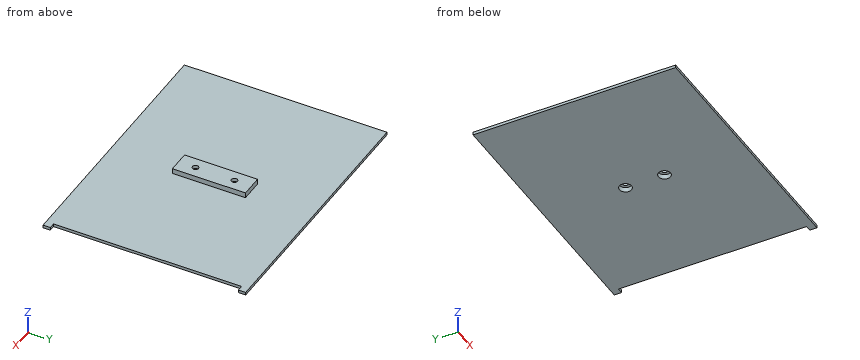
```python
from build123d import *

# Parameters (mm, degrees)
EXTRUDE_2_DEPTH     = 1.5
SKETCH_2_W          = 11.5
SKETCH_2_H          = 37.5
EXTRUDE_3_DEPTH     = 2.7
SKETCH_3_R          = 3.1
CUT_EXTRUDE_1_DEPTH = 2.5
SKETCH_4_R          = 1.55
CUT_EXTRUDE_2_DEPTH = 2.5


with BuildPart() as part:
    # Эскиз1 → Бобышка-Вытянуть2 (new body)
    with BuildSketch(Plane.XY):
        Polygon((-67, -52), (67, -52), (67, -48.25), (64, -48.25), (64, 48.25), (67, 48.25), (67, 52), (-67, 52), align=None)
    extrude(amount=EXTRUDE_2_DEPTH)

    # Эскиз2 → Бобышка-Вытянуть3 (add)
    with BuildSketch(Plane.XY.offset(1.5)):
        Rectangle(SKETCH_2_W, SKETCH_2_H)
    extrude(amount=EXTRUDE_3_DEPTH)

    # Эскиз3 → Вырез-Вытянуть1 (cut)
    with BuildSketch(Plane(origin=(0, 0, 0), x_dir=(-1, 0, 0), z_dir=(0, 0, -1))):
        with Locations((0, -10)):
            Circle(SKETCH_3_R)
        with Locations((0, 10)):
            Circle(SKETCH_3_R)
    extrude(amount=-CUT_EXTRUDE_1_DEPTH, mode=Mode.SUBTRACT)

    # Эскиз4 → Вырез-Вытянуть2 (cut)
    with BuildSketch(Plane(origin=(0, 0, 2.5), x_dir=(-1, 0, 0), z_dir=(0, 0, -1))):
        with Locations((0, -10)):
            Circle(SKETCH_4_R)
        with Locations((0, 10)):
            Circle(SKETCH_4_R)
    extrude(amount=-CUT_EXTRUDE_2_DEPTH, mode=Mode.SUBTRACT)


solid = part.part
```
Check sheet for the modelled part. Datum: model origin and axes. Units: mm. Round coordinates to 2 decimals unless told otherwise and drop trailing zeros. Order: outer loops, then holes, each group sorted by start corner. A loop starts at its lowest first (then second) coordinate and runs counter-clockwise, first axis right, second up. Notation, with made-up numbers: (-9.75, -31) -> (11.25, -31) arc R11 cw to (11.25, -16) -> close; hole circle Ø11 at (-12, -21.5). An arc over 180 degrees is marked (long way). One line per item, written item: value. Start each with the question number.
Q1. Cross-section at B-B (x = 0). Record the boundary of the cut face in (y, z).
Q2. Cross-section at D-D (x = 16.5). Record the boundary of the cut face in (y, z), and give its area (3 significant figures).
Q3. Gauge pin test, flat ends, axial feed: pin 1 Ø1.4 at (x, z) = (-1.5, 3.5) entering from -Y; pin 2 Ø2 at (x, z) = (-2.5, 3.5) entering from +Y; pin 3 Ø8 at (x, y) = (-45, 5) entering from +Z. Record the tip position at first contact, or that the pin passes through.
Q4. Thickness scan on line 1 (Y direction, x = 0, z = 3.1); line 2 (Y direction, x = 0, z = 0.8); line 3 (Z direction, x = 12, y = -19.5). Record the ranges inside material, lowest first.
Q5. Cross-section at C-C (z = 0.65). Record the boundary of the cut face in (x, y).
Q6. Cross-section at A-A (y = 10). Record the boundary of the cut face in (x, z), and give its area (3 significant figures).
Completed:
1. outline: (-52, 0) -> (-13.1, 0) -> (-13.1, 2.5) -> (-11.55, 2.5) -> (-11.55, 4.2) -> (-18.75, 4.2) -> (-18.75, 1.5) -> (-52, 1.5) -> close; (-8.45, 2.5) -> (-6.9, 2.5) -> (-6.9, 0) -> (6.9, 0) -> (6.9, 2.5) -> (8.45, 2.5) -> (8.45, 4.2) -> (-8.45, 4.2) -> close; (11.55, 2.5) -> (13.1, 2.5) -> (13.1, 0) -> (52, 0) -> (52, 1.5) -> (18.75, 1.5) -> (18.75, 4.2) -> (11.55, 4.2) -> close
2. outline: (-52, 0) -> (52, 0) -> (52, 1.5) -> (-52, 1.5) -> close
2. area: 156 mm²
3. pin 1: stops at y = -18.75
3. pin 2: stops at y = 18.75
3. pin 3: stops at z = 1.5
4. line 1: y = -18.75 to -11.55, -8.45 to 8.45, 11.55 to 18.75
4. line 2: y = -52 to -13.1, -6.9 to 6.9, 13.1 to 52
4. line 3: z = 0 to 1.5
5. outline: (-67, -52) -> (67, -52) -> (67, -48.25) -> (64, -48.25) -> (64, 48.25) -> (67, 48.25) -> (67, 52) -> (-67, 52) -> close; hole circle Ø6.2 at (0, -10); hole circle Ø6.2 at (0, 10)
6. outline: (-67, 0) -> (-3.1, 0) -> (-3.1, 2.5) -> (-1.55, 2.5) -> (-1.55, 4.2) -> (-5.75, 4.2) -> (-5.75, 1.5) -> (-67, 1.5) -> close; (1.55, 2.5) -> (3.1, 2.5) -> (3.1, 0) -> (64, 0) -> (64, 1.5) -> (5.75, 1.5) -> (5.75, 4.2) -> (1.55, 4.2) -> close
6. area: 207 mm²
